Work out the finished part from the listing and answer in its coordinate system (mm). A direction names the side the tool comes from. Give positions to 0.01 mm unless a question says otherwise; leave off trailing zeros. Order: outer loops, then holes, each group sorted by start corner. A loop starts at its lowest first (then second) coordinate and runs counter-clockwise, first axis right, second up. Notation, with made-up numbers: (26, -5) -> (34, -5) arc R25 cw to (34, 18) -> close; hole circle Ø8 at (-7.75, 45). An arc over 180 degrees is marked (long way). Use a Markdown table: item, result. Add a question column.
```python
from build123d import *

# Parameters (mm, degrees)
BOX003_W        = 40
BOX003_H        = 70
BOX003_DEPTH    = 24
SKETCH012_R     = 2.2
SKETCH012_W     = 28
SKETCH012_H     = 35
POCKET012_DEPTH = 37
CHAMFER004_SIZE = 7
SKETCH013_R     = 3.75
POCKET013_DEPTH = 8
SKETCH014_R     = 1.45
POCKET014_DEPTH = 25


with BuildPart() as part:
    # Box003 → Box003 (new body)
    with BuildSketch(Plane(origin=(-267, 176.2, 345), x_dir=(1, 0, 0), z_dir=(0, 0, 1))):
        with Locations((20, 35)):
            Rectangle(BOX003_W, BOX003_H)
    extrude(amount=BOX003_DEPTH)

    # Sketch012 → Pocket012 (cut)
    with BuildSketch(Plane(origin=(-267, 176.2, 369), x_dir=(1, 0, 0), z_dir=(0, 0, 1))):
        with Locations((14, 60)):
            Circle(SKETCH012_R)
        with Locations((14, 10)):
            Circle(SKETCH012_R)
        with Locations((14, 35)):
            Rectangle(SKETCH012_W, SKETCH012_H)
    extrude(amount=-POCKET012_DEPTH, mode=Mode.SUBTRACT)

    # Chamfer004
    chamfer004_edges = [part.edges().sort_by_distance(p)[0] for p in [
        (-227, 176.2, 357),
        (-267, 176.2, 357),
        (-267, 193.7, 357),
        (-239, 193.7, 357),
        (-239, 228.7, 357),
        (-267, 228.7, 357),
        (-267, 246.2, 357),
        (-227, 246.2, 357),
    ]]
    chamfer(chamfer004_edges, length=CHAMFER004_SIZE)

    # Sketch013 → Pocket013 (cut)
    with BuildSketch(Plane(origin=(-267, 176.2, 369), x_dir=(1, 0, 0), z_dir=(0, 0, 1))):
        with Locations((14, 60)):
            Circle(SKETCH013_R)
        with Locations((14, 10)):
            Circle(SKETCH013_R)
    extrude(amount=-POCKET013_DEPTH, mode=Mode.SUBTRACT)

    # Sketch014 → Pocket014 (cut)
    with BuildSketch(Plane(origin=(-227, 176.2, 345), x_dir=(0, 1, 0), z_dir=(1, 0, 0))):
        with Locations((13.75, 9)):
            Circle(SKETCH014_R)
        with Locations((56.25, 9)):
            Circle(SKETCH014_R)
    extrude(amount=-POCKET014_DEPTH, mode=Mode.SUBTRACT)


solid = part.part
```
1) The part is cut by section D-D, the plane x = -257.5. Determine the outline of the cut face in (y, z), then the cut area to 3 significant figures.
2) The part is cut by section B-B, the plane z = 354. Determine the outline of the cut face in (x, y), then the cut area to 3 significant figures.
3) The part is cut by section A-A, the plane x = -263.5. Determine the outline of the cut face in (y, z), then the cut area to 3 significant figures.
4) Which of the six approach directions +Z, -Z, +X, -X, +Y, -Y give full straight-line access (tool end or side, diameter ignored) to faces 1 (the flat face through (-267, 185, 357)), 2 (the cylindrical face through (-249.423, 187.326, 365.056)), 3 (the flat face through (-252, 232, 354)), 4 (the flat face through (-242.5, 197.2, 357.2))?
5) Flat-ended cylindrical pins translate along their axes: pin 1 (1.7 mm diameter, centred on y = 189.95, z = 354, fed in from +X); pin 2 (2 mm diameter, centred on x = -254.5, y = 187, fed in from +Z); pin 3 (1.5 mm diameter, centred on y = 219, z = 356.5, fed in from -X). Find the tip coordinate at first contact, or state that the pin passes through.
6) Determine the mould class of faces 5 (the flat face through (-252, 190, 354)), 6 (the flat face through (-227, 211, 357)), 7 (the flat face through (-263.5, 179.7, 356.8)), 8 (the flat face through (-230.5, 242.7, 356.8)) for opening direction Y: released by +Y, released by -Y, zero draft, split by the parting line, or undercut.
7) The part is cut by section C-C, the plane x = -253. Determine the outline of the cut face in (y, z).
8) Straight lines are drawn through the part: line 1 (Y direction, x = -253, z = 362.75); line 2 (Y direction, x = -253, z = 357.75); line 3 (X direction, y = 186.2, z = 365.5). For each, find the intervals that lie inside material, in ascending order.
A:
| question | item | result |
|---|---|---|
| 1 | outline | (176.2, 345) -> (193.7, 345) -> (193.7, 369) -> (176.2, 369) -> close; (228.7, 345) -> (246.2, 345) -> (246.2, 369) -> (228.7, 369) -> close |
| 1 | area | 840 mm^2 |
| 2 | outline | (-267, 183.2) -> (-260, 176.2) -> (-234, 176.2) -> (-227, 183.2) -> (-227, 188.5) -> (-252, 188.5) -> (-252, 191.4) -> (-227, 191.4) -> (-227, 231) -> (-252, 231) -> (-252, 233.9) -> (-227, 233.9) -> (-227, 239.2) -> (-234, 246.2) -> (-260, 246.2) -> (-267, 239.2) -> (-267, 235.7) -> (-260, 228.7) -> (-246, 228.7) -> (-239, 221.7) -> (-239, 200.7) -> (-246, 193.7) -> (-260, 193.7) -> (-267, 186.7) -> close; hole circle Ø4.4 at (-253, 186.2); hole circle Ø4.4 at (-253, 236.2) |
| 2 | area | 1,550 mm^2 |
| 3 | outline | (179.7, 345) -> (190.2, 345) -> (190.2, 369) -> (179.7, 369) -> close; (232.2, 345) -> (242.7, 345) -> (242.7, 369) -> (232.2, 369) -> close |
| 3 | area | 504 mm^2 |
| 4 | face 1 | +Z, -Z, -X, +Y, -Y |
| 4 | face 2 | +Z |
| 4 | face 3 | +X |
| 4 | face 4 | +Z, -Z, -X |
| 5 | pin 1 | x = -252 |
| 5 | pin 2 | z = 361 |
| 5 | pin 3 | x = -239 |
| 6 | face 5 | undercut |
| 6 | face 6 | zero draft |
| 6 | face 7 | released by -Y |
| 6 | face 8 | released by +Y |
| 7 | outline | (176.2, 345) -> (184, 345) -> (184, 361) -> (182.45, 361) -> (182.45, 369) -> (176.2, 369) -> close; (188.4, 345) -> (193.7, 345) -> (193.7, 369) -> (189.95, 369) -> (189.95, 361) -> (188.4, 361) -> close; (228.7, 345) -> (234, 345) -> (234, 361) -> (232.45, 361) -> (232.45, 369) -> (228.7, 369) -> close; (238.4, 345) -> (246.2, 345) -> (246.2, 369) -> (239.95, 369) -> (239.95, 361) -> (238.4, 361) -> close |
| 8 | line 1 | 176.2 to 182.45, 189.95 to 193.7, 228.7 to 232.45, 239.95 to 246.2 |
| 8 | line 2 | 176.2 to 184, 188.4 to 193.7, 228.7 to 234, 238.4 to 246.2 |
| 8 | line 3 | -267 to -256.75, -249.25 to -227 |
